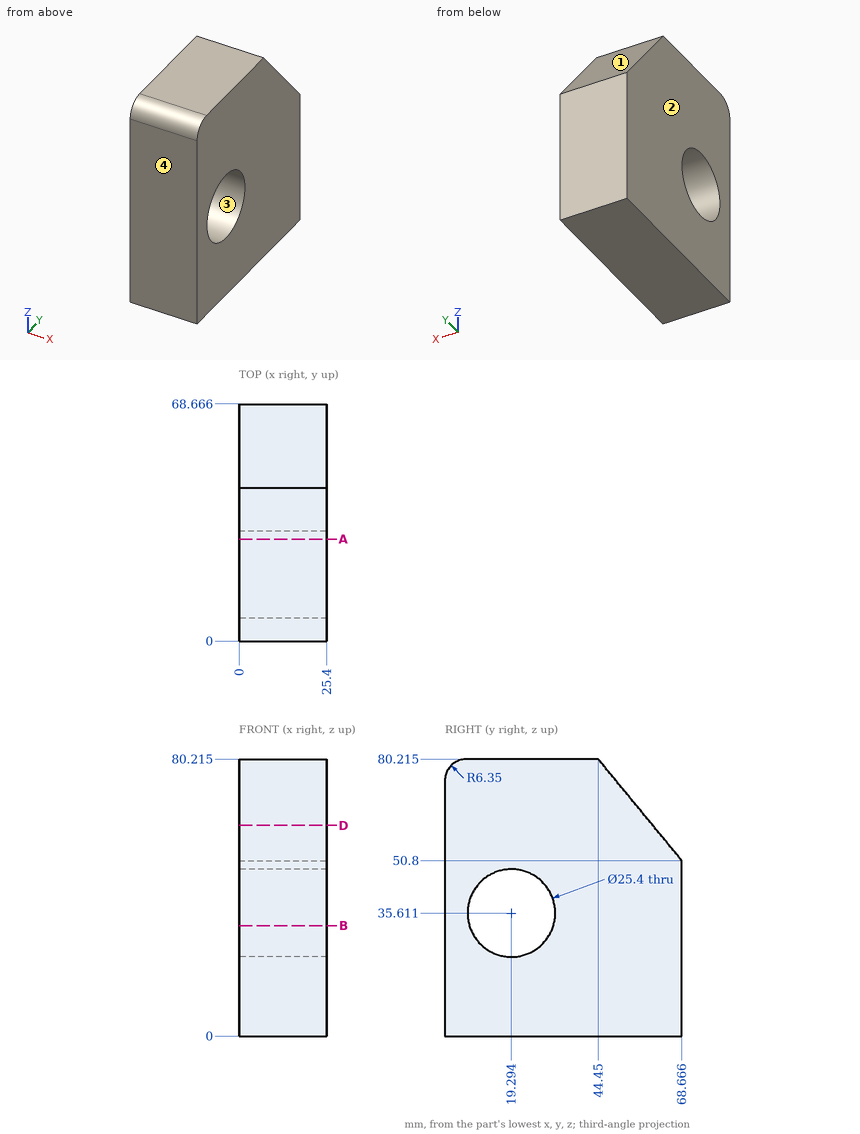
For this review, use the dimensioned drawing (mm, ordinates from the lowest corner) and the shaded views. Coordinates: 2 decimals unless noted, no trailing zeros. Loops run counter-clockwise (first coordinate to the right, second up) from the corner with the lowest first, then second, coordinate; pieces in that order, holes last. Notation, with made-up numbers: (16, -32.75) -> (54, -32.75) arc R15 cw to (54, -26.75) -> close; hole circle Ø7 at (22, 68). An arc over 180 degrees is marked (long way). Use a Markdown table: item, result. Add a question column.
Item 1: We need section A-A, the plane y = 29.5. Write out the cut boundary in (x, z) (1 decimal), and give its area (3 significant figures).
Item 2: The part is to be moulded in two halves that separate along Y. For the marked faces 1, 2, 3 and 4, say which applies: +Y half, -Y half, draft (parallel to the pull), parting line (faces both ways), or undercut.
Item 3: We need section D-D, the plane z = 61. Write out the cut boundary in (x, y).
Item 4: Clearance check with a flat-ended pin moving along its axis: P1, Ø4, axis at x = 13.5, y = 59.5, coming from the +Z side (1 decimal). State where the tip first meets the part, or that it passes through.
Item 5: We need section B-B, the plane z = 32. Write out the cut boundary in (x, y) (1 decimal).
Item 6: Wall thickness on L1, parallel to Y at x = 14.5, z = 25.5 (1 decimal); L2, parallel to Y at x = 14.5, z = 34.5 (1 decimal); L3, parallel to Z at x = 10, y = 27 (1 decimal): over which ranges is each line inside the solid? List them lowest first. Write a range as from..to.
Numbers:
| question | item | result |
|---|---|---|
| 1 | outline | (0, 0) -> (25.4, 0) -> (25.4, 28.1) -> (0, 28.1) -> close; (0, 43.2) -> (25.4, 43.2) -> (25.4, 80.2) -> (0, 80.2) -> close |
| 1 | area | 1,650 mm^2 |
| 2 | face 1 | +Y half |
| 2 | face 2 | draft |
| 2 | face 3 | undercut |
| 2 | face 4 | -Y half |
| 3 | outline | (0, 0) -> (25.4, 0) -> (25.4, 60.27) -> (0, 60.27) -> close |
| 4 | P1 | stops at z = 64.4 |
| 5 | outline | (0, 0) -> (25.4, 0) -> (25.4, 7.1) -> (0, 7.1) -> close; (0, 31.5) -> (25.4, 31.5) -> (25.4, 68.7) -> (0, 68.7) -> close |
| 6 | L1 | y = 0..11.6, 27..68.7 |
| 6 | L2 | y = 0..6.6, 31.9..68.7 |
| 6 | L3 | z = 0..25.5, 45.7..80.2 |
